```python
from build123d import *

# Parameters (mm, degrees)
F0_W      = 45
F0_H      = 100
F1_DEPTH  = 10.2
F2_W      = 17
F2_H      = 70
F3_DEPTH  = 8.6
F4_W      = 41.8
F4_H      = 100
F5_DEPTH  = 7
F8_R      = 16.5
F9_DEPTH  = 10
F14_W     = 131.8
F14_H     = 10.2
F15_DEPTH = 0.8


with BuildPart() as f1:
    # F0 (on Top) → F1 (new body)
    with BuildSketch(Plane.XY):
        with Locations((-33.8353561237, -14.8088461805)):
            Rectangle(F0_W, F0_H)
    extrude(amount=F1_DEPTH)

    # F2 (on face) → F3 (cut)
    with BuildSketch(Plane.XY.offset(10.2)):
        with Locations((-33.8353561237, -29.8088461805)):
            Rectangle(F2_W, F2_H)
    extrude(amount=-F3_DEPTH, mode=Mode.SUBTRACT)


with BuildPart() as f5:
    # F4 (on Top) → F5 (new body)
    with BuildSketch(Plane.XY):
        with Locations((-35.4353561237, -14.8088461805)):
            Rectangle(F4_W, F4_H)
    extrude(amount=F5_DEPTH)


with BuildPart() as f5_1:
    # F6: moved
    add(f5.part.moved(Location((1.6, 0, 1.6))))


with BuildPart() as f1_1:
    add(f1.part)

    # F7: cut F5
    add(f5_1.part, mode=Mode.SUBTRACT)


with BuildPart() as f9:
    # F8 (on Top) → F9 (new body)
    with BuildSketch(Plane.XY):
        with Locations((-33.8353561237, -64.8088461805)):
            Circle(F8_R)
    extrude(amount=F9_DEPTH)


with BuildPart() as f9_1:
    # F10: moved
    add(f9.part.moved(Location((0, 75, 4))))


with BuildPart() as f1_2:
    add(f1_1.part)

    # F11: cut F9
    add(f9_1.part, mode=Mode.SUBTRACT)


with BuildPart() as f12_1:
    # F12: copy of F1
    add(f1_2.part.moved(Location((43.4, 0, 0))))


with BuildPart() as f13_1:
    # F13: copy of F12_1
    add(f12_1.part.moved(Location((43.4, 0, 0))))


with BuildPart() as f1_3:
    add(f1_2.part)

    add(f12_1.part)  # F15 merges F12_1

    add(f13_1.part)  # F15 merges F13_1
    # F14 (on face) → F15 (join)
    with BuildSketch(Plane(origin=(0, 35.1911538195, 0), x_dir=(-1, 0, 0), z_dir=(0, 1, 0))):
        with Locations((-9.5646438763, 5.1)):
            Rectangle(F14_W, F14_H)
    extrude(amount=-F15_DEPTH)


solid = f1_3.part
```
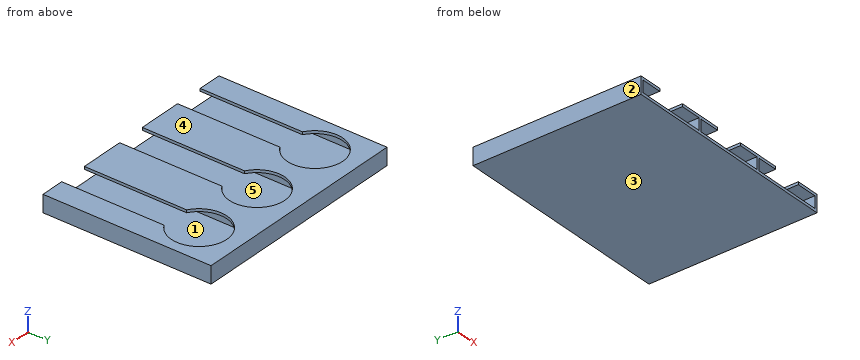
Source: CAD feature listing. Evaluate the final solid. Frame: model axes, mm. Face numbers are marked on the shaded views. A direction names the side the tool comes from. Round coordinates to 2 decimals unless told otherwise and drop trailing zeros. Loops run counter-clockwise (first coordinate to the right, second up) from the corner with the lowest first, then second, coordinate; pieces in that order, holes last. Notation, with made-up numbers: M -30.5,22 L 27.5,22 A20 cw 27.5,57 Z; hole C 11.5,71 d1. An arc over 180 degrees is marked long. Put each result on its own line as item: value.
(1) Section B-B, the plane z = 6.5. Return loops of the section in (x, y).
Solutions:
outline: M -56.34,-64.81 L -54.74,-64.81 L -54.74,34.39 L -12.94,34.39 L -12.94,-64.81 L -11.34,-64.81 L -11.34,34.39 L 30.46,34.39 L 30.46,-64.81 L 32.06,-64.81 L 32.06,34.39 L 73.86,34.39 L 73.86,-64.81 L 75.46,-64.81 L 75.46,35.19 L -56.34,35.19 Z
(2) Section A-A, the plane x = -44. Return loops of the section in (y, z).
Solutions:
outline: M -64.81,0 L 35.19,0 L 35.19,10.2 L 23.19,10.2 L 23.19,8.6 L 34.39,8.6 L 34.39,1.6 L -64.81,1.6 Z; M -64.81,8.6 L -2.81,8.6 L -2.81,10.2 L -64.81,10.2 Z
(3) Ray query, line 1 (X direction, y = -41, z = 5); line 2 (X direction, y = 9.5, z = 8.75); line 3 (Z direction, x = -2, y = -26). Return the intervals inside material, ascending. Write a range as [from, to].
Solutions:
line 1: [-56.34, -54.74], [-12.94, -11.34], [30.46, 32.06], [73.86, 75.46]
line 2: [-56.34, -50.32], [-17.35, -6.92], [26.05, 36.48], [69.45, 75.46]
line 3: [0, 1.6], [8.6, 10.2]
(4) Section D-D, the plane x = 10.5. Return loops of the section in (y, z), and give its area (3 significant figures).
Solutions:
outline: M -64.81,0 L 35.19,0 L 35.19,10.2 L 26.66,10.2 L 26.66,8.6 L 34.39,8.6 L 34.39,1.6 L -64.81,1.6 Z
area: 179 mm²
(5) First-contact query: pin 1 (12.5 mm diameter, centred on x = -37.5, y = 7, fed in from +Z); pin 2 (5.5 mm diameter, centred on x = 61.5, z = 4.5, fed in from -Y). Flat tips, straight axial feed; report the tip coordinate or a pass-through.
Solutions:
pin 1: z = 1.6
pin 2: y = 34.39
(6) Pull-direction query (Z, two-part tool) for the marked faces 3, 4 and 5; classes: released by +Z, released by -Z, zero draft, split by the parting line, or undercut.
Solutions:
face 3: released by -Z
face 4: released by +Z
face 5: undercut
(7) Access query for the marked faces 1 and 2. Directions: +Z, -Z, +X, -X, +Y, -Y. A direction counts if a zero-diameter tool reaches every point of the face in a straight line with its end or side. Return the directions, or none.
Solutions:
face 1: -Y
face 2: +Z, -Z, -X, +Y, -Y
(8) Section C-C, the plane y = -37. Return loops of the section in (x, z).
Solutions:
outline: M -56.34,0 L 75.46,0 L 75.46,10.2 L 61.46,10.2 L 61.46,8.6 L 73.86,8.6 L 73.86,1.6 L 32.06,1.6 L 32.06,8.6 L 44.46,8.6 L 44.46,10.2 L 18.06,10.2 L 18.06,8.6 L 30.46,8.6 L 30.46,1.6 L -11.34,1.6 L -11.34,8.6 L 1.06,8.6 L 1.06,10.2 L -25.34,10.2 L -25.34,8.6 L -12.94,8.6 L -12.94,1.6 L -54.74,1.6 L -54.74,8.6 L -42.34,8.6 L -42.34,10.2 L -56.34,10.2 Z
